The drawing under review shows one solid part. Ordinate dimensions are in mm from its lowest x, y, z. Round coordinates to 2 decimals unless told otherwise and drop trailing zeros. Order: outer loops, then holes, each group sorted by start corner. A loop starts at its lowest first (then second) coordinate and runs counter-clockwise, first axis right, second up. Notation, with made-up numbers: M 51.5,14 L 110.5,14 A29 cw 110.5,45 Z; hole C -2,30.5 d6. An arc over 180 degrees is marked long. Use a Markdown table: item, result.
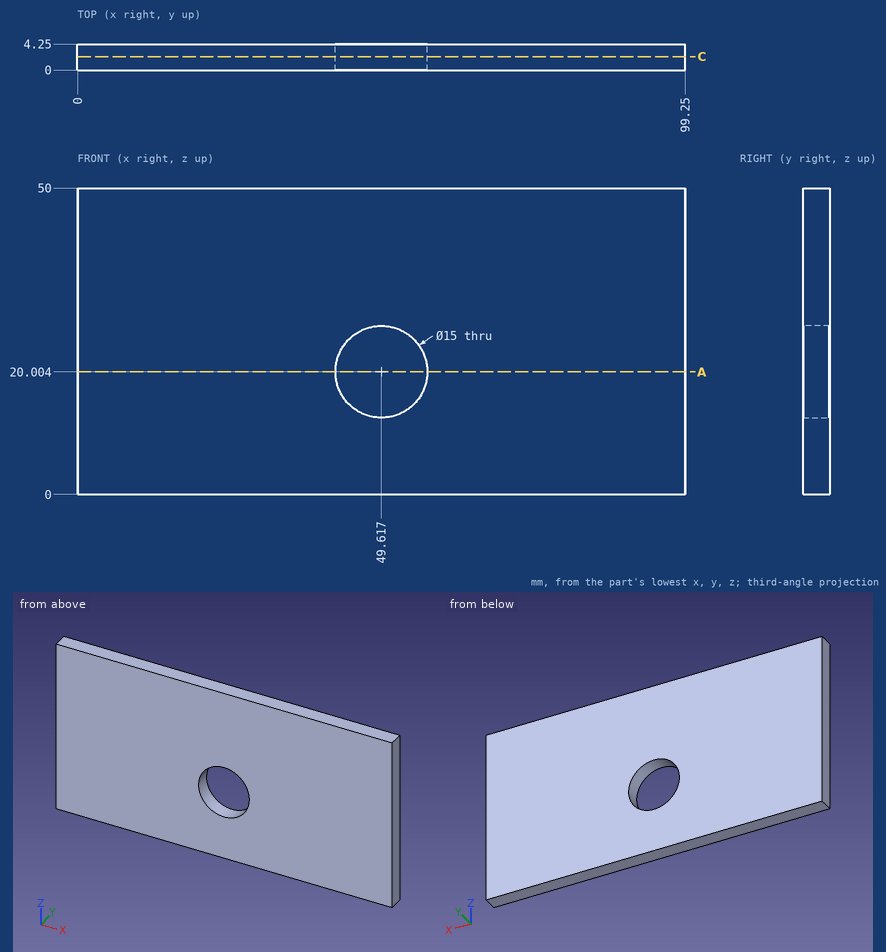
Q1. Wall thickness on line 1 along Z through (x, y) = (52, 3.6) (1 decimal): over which ranges is the line inside the solid? List them lowest first. Write a range as [from, to].
Determined:
| item | result |
|---|---|
| line 1 | z = [0, 12.9], [27.1, 50] |
Q2. Add section C-C (y = 2.2). Write out the cut boundary in (x, z).
Determined:
| item | result |
|---|---|
| outline | M 0,0 L 99.25,0 L 99.25,50 L 0,50 Z; hole C 49.62,20 d15 |
Q3. Clearance check with flat-ended pins moving along their axes: pin 1 (2 mm diameter, centred on x = 42, z = 38.5, fed in from -Y); pin 2 (13.5 mm diameter, centred on x = 49.62, z = 20, fed in from -Y). State where each tip first meets the part, or that it passes through.
Determined:
| item | result |
|---|---|
| pin 1 | stops at y = 0 |
| pin 2 | passes through |
Q4. Add section A-A (z = 20). Write out the cut boundary in (x, y).
Determined:
| item | result |
|---|---|
| outline | M 0,0 L 42.12,0 L 42.12,4.25 L 0,4.25 Z; M 57.12,0 L 99.25,0 L 99.25,4.25 L 57.12,4.25 Z |
